Input: part model. Units: mm. Frame: model coordinates. A direction names the side the tool comes from. Round coordinates to 2 decimals unless told otherwise and drop trailing zeros. Order: outer loops, then holes, each group sorted by start corner. A loop starts at its lowest first (then second) coordinate and runs counter-clockwise, first axis right, second up. Notation, with made-up numbers: (35.25, -28) -> (41.25, -28) arc R17 cw to (41.25, -5) -> close; hole circle Ø5 at (-37, 26). An arc over 180 degrees is marked (long way). Use a Markdown table: item, result.
from build123d import *

# Parameters (mm, degrees)
CUT_EXTRUDE1_DEPTH      = 74.218850032
CUT_EXTRUDE1_DEPTH_BACK = 74.218850032
SKETCH2_R               = 1.75
CHAMFER1_SIZE           = 2


with BuildPart() as part:
    # Sketch1 → Revolve1 (revolve)
    with BuildSketch(Plane(origin=(0, 0, 0), x_dir=(0, 0, -1), z_dir=(1, 0, 0))):
        Polygon((-10, 14), (-10, 4), (-49, 4), (-50, 3), (-50, 1), (-49, 0), (-19, 0), (-18, -1), (-18, -14), (-17, -15), (-15.25, -15), (-14.25, -14), (-14.25, -5.1), (-14.15, -5), (-11.75, -5), (-6.75, 0), (-6.75, 14), (-7.75, 15), (-9, 15), align=None)
    revolve(axis=Axis((0, 143.307692308, 0), (0, -1, 0)))

    # Sketch2 → Cut-Extrude1 (cut, two sides: drawn at the far end of the back side and taken through both)
    with BuildSketch(Plane(origin=(0, 4, 0), x_dir=(1, 0, 0), z_dir=(0, 1, 0)).offset(-CUT_EXTRUDE1_DEPTH_BACK)):
        with Locations(Location((0, 37.5, 0), (0, 0, 270))):
            Circle(SKETCH2_R)
        with Locations(Location((26.516504294, 26.516504294, 0), (0, 0, 270))):
            Circle(SKETCH2_R)
        with Locations(Location((37.5, 0, 0), (0, 0, 270))):
            Circle(SKETCH2_R)
        with Locations(Location((26.516504294, -26.516504294, 0), (0, 0, 270))):
            Circle(SKETCH2_R)
        with Locations(Location((0, -37.5, 0), (0, 0, 270))):
            Circle(SKETCH2_R)
        with Locations(Location((-26.516504294, -26.516504294, 0), (0, 0, 270))):
            Circle(SKETCH2_R)
        with Locations(Location((-37.5, 0, 0), (0, 0, 270))):
            Circle(SKETCH2_R)
        with Locations(Location((-26.516504294, 26.516504294, 0), (0, 0, 270))):
            Circle(SKETCH2_R)
    extrude(amount=CUT_EXTRUDE1_DEPTH + CUT_EXTRUDE1_DEPTH_BACK, mode=Mode.SUBTRACT)

    # Chamfer1
    chamfer1_edges = [part.edges().sort_by_distance(p)[0] for p in [
        (0, 0, -39.25),
        (26.516504294, 0, -28.266504294),
        (37.5, 0, -1.75),
        (26.516504294, 0, 24.766504294),
        (0, 0, 35.75),
        (-26.516504294, 0, 24.766504294),
        (-37.5, 0, -1.75),
        (-26.516504294, 0, -28.266504294),
    ]]
    chamfer(chamfer1_edges, length=CHAMFER1_SIZE)


solid = part.part
1) Cut plane D-D on y = 8. Return loops of the section in (x, z), and give its area (3 significant figures).
Results found:
| item | result |
|---|---|
| outline | circle Ø20 at (0, 0); hole circle Ø13.5 at (0, 0) |
| area | 171 mm² |
2) Set-up query: faces 1 (the cylindrical face through (5.458, -9.488, 13.163)), 2 (the cylindrical face through (9.76, 8.93, -2.17)), 3 (the cylindrical face through (-25.334, 2.986, -27.806)). Return all of +Z, -Z, +X, -X, +Y, -Y with unobstructed straight access to the full face (end or side cutting, diameter ignored); none if empty.
Results found:
| item | result |
|---|---|
| face 1 | -Y |
| face 2 | +Y |
| face 3 | +Y, -Y |
3) Pull-direction query (Z, two-part tool) for faces 4 (the flat face through (-1, 0, 21)), 5 (the flat face through (-12, -5, 2)), 6 (the cylindrical face through (-15.02, 1.99, 47.69)); classes: +Z half, -Z half, draft (parallel to the pull), parting line (faces both ways), or undercut.
Results found:
| item | result |
|---|---|
| face 4 | draft |
| face 5 | undercut |
| face 6 | parting line |
4) Line query: L1, parallel to Z at x = 0, y = 7.5; L2, parallel to Z at x = 0, y = -7.25; L3, parallel to Z at x = 0, y = 3.6. Output: solid intervals per line, ascending. Write a range as [from, to].
Results found:
| item | result |
|---|---|
| L1 | z = [-10, -6.75], [6.75, 10] |
| L2 | z = [-18, -14.25], [14.25, 18] |
| L3 | z = [-49.4, -39.25], [-35.75, -6.75], [6.75, 35.75], [39.25, 49.4] |
5) Cut plane A-A on y = -10.25. Return loops of the section in (x, z).
Results found:
| item | result |
|---|---|
| outline | circle Ø36 at (0, 0); hole circle Ø28.5 at (0, 0) |
6) Cut plane B-B on z = 0. Count the separate pieces of the cut face and the enclosed holes in it, and give its area (3 significant figures).
Results found:
| item | result |
|---|---|
| separate pieces | 4 |
| enclosed holes | 0 |
| area | 539 mm² |
7) Pin query (flat end, axial travel): pin 1 Ø4 at (x, z) = (0, -37.5) entering from -Y; pin 2 Ø11 at (x, z) = (0, 0) entering from +Y; pin 3 Ø1 at (x, y) = (27.5, 3) entering from -Z; pin 4 Ø4 at (y, z) = (1, 16.5) entering from -X. Return the tip coordinate at first contact, or that it passes through.
Results found:
| item | result |
|---|---|
| pin 1 | stops at y = 1.75 |
| pin 2 | passes through |
| pin 3 | stops at z = -42.08 |
| pin 4 | stops at x = -47.85 |
